```python
from build123d import *

# Parameters (mm, degrees)
BOSS_EXTRUDE1_DEPTH     = 50
CUT_EXTRUDE1_DEPTH      = 100
CUT_EXTRUDE1_DEPTH_BACK = 100
SKETCH2_R               = 2
SKETCH3_W               = 56
SKETCH3_H               = 15
BOSS_EXTRUDE2_DEPTH     = 3


with BuildPart() as part:
    # Sketch1 → Boss-Extrude1 (new, symmetric)
    with BuildSketch(Plane.XY):
        with BuildLine():
            Line((-28, 25), (-28, -10))
            Line((-28, -10), (-25, -10))
            Line((-25, -10), (-25, 0))
            Line((-25, 0), (-20, 0))
            ThreePointArc((-20, 0), (0, 20), (20, 0))
            Line((20, 0), (25, 0))
            Line((25, 0), (25, -10))
            Line((25, -10), (28, -10))
            Line((28, -10), (28, 25))
            Line((28, 25), (-28, 25))
        make_face()
    extrude(amount=BOSS_EXTRUDE1_DEPTH, both=True)

    # Sketch2 → Cut-Extrude1 (cut, two sides: drawn at the far end of the back side and taken through both)
    with BuildSketch(Plane(origin=(-25, 0, 0), x_dir=(0, 0, -1), z_dir=(1, 0, 0)).offset(-CUT_EXTRUDE1_DEPTH_BACK)):
        with Locations((-40, -5)):
            Circle(SKETCH2_R)
        with Locations((0, -5)):
            Circle(SKETCH2_R)
        with Locations((40, -5)):
            Circle(SKETCH2_R)
    extrude(amount=CUT_EXTRUDE1_DEPTH + CUT_EXTRUDE1_DEPTH_BACK, mode=Mode.SUBTRACT)

    # Sketch3 → Boss-Extrude2 (add)
    with BuildSketch(Plane.XY.offset(50)):
        with Locations((0, 17.5)):
            Rectangle(SKETCH3_W, SKETCH3_H)
    boss_extrude2 = extrude(amount=BOSS_EXTRUDE2_DEPTH)

    # Mirror1: Boss-Extrude2 across plane
    add(boss_extrude2.mirror(Plane.XY))


solid = part.part
```
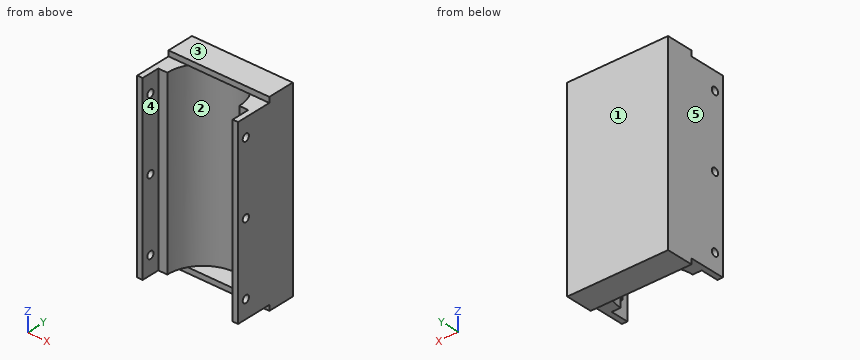
Geometry check sheet. Reference: the model listing, model coordinates, mm. Face numbers are marked on the shaded views. A direction names the side the tool comes from. Give positions to 0.01 mm unless a question says otherwise; leave off trailing zeros. Order: outer loops, then holes, each group sorted by start corner. A loop starts at its lowest first (then second) coordinate and runs counter-clockwise, first axis right, second up. Notation, with made-up numbers: (20, -8.5) - (68, -8.5) arc R27 cw to (68, 12.5) - close; hole circle Ø10 at (-4, 13.5). An arc over 180 degrees is marked (long way). Write item = value, one per line. Start each with the question number.
1) Section check A-A (z = 0). Enter the section's corners in (x, y), then the cut area to 3 significant figures.
2) Section check C-C (x = 23). Enter the section's corners in (y, z).
3) Gauge pin test, flat ends, axial feed: pin 1 Ø11.5 at (x, y) = (23.5, 2.5) entering from -Z; pin 2 Ø3.5 at (x, z) = (5, -52) entering from -Y; pin 3 Ø6.5 at (y, z) = (-5, -40) entering from +X; pin 4 Ø4 at (x, z) = (22, 12.5) entering from -Y. Record the tip position at first contact, or that the pin passes through.
4) Draft check along Z on the marked faces 1, 2 and 3. Enter one of: released by +Z, released by -Z, zero draft, split by the parting line, or undercut.
5) Section check D-D (y = 18.5). Enter the section's corners in (x, z), then the cut area to 3 significant figures.
6) Scan lines: L1, parallel to Z at x = 26.4, y = -5; L2, parallel to X at y = -1, z = 15; L3, parallel to Y at x = -27, z = 40. Record each from-to range of solid material in increasing order.
7) Access from +Z, -Z, +X, -X, +Y, -Y to the whole of each face (thin tool, end or side, straight path). Record for the marked faces 4 and 5.
8) Section check B-B (y = 7). Enter the section's corners in (x, z) (3 decimals), then the cut area to 3 significant figures.
Geometry check:
q1.outline = (-28, -10) - (-25, -10) - (-25, -7) - (-28, -7) - close; (-28, -3) - (-25, -3) - (-25, 0) - (-20, 0) arc R20 cw to (20, 0) - (25, 0) - (25, -3) - (28, -3) - (28, 25) - (-28, 25) - close; (25, -10) - (28, -10) - (28, -7) - (25, -7) - close
q1.area = 808 mm2
q2.outline = (0, -50) - (10, -50) - (10, -53) - (25, -53) - (25, 53) - (10, 53) - (10, 50) - (0, 50) - close
q3.pin_1 = -50
q3.pin_2 = 10
q3.pin_3 = 28
q3.pin_4 = 0
q4.face_1 = zero draft
q4.face_2 = undercut
q4.face_3 = released by +Z
q5.outline = (-28, -53) - (28, -53) - (28, 53) - (-28, 53) - close; hole (-7.6, -50) - (7.6, -50) - (7.6, 50) - (-7.6, 50) - close
q5.area = 4,420 mm2
q6.L1 = -50 to -42, -38 to -2, 2 to 38, 42 to 50
q6.L2 = -28 to -25, 25 to 28
q6.L3 = -10 to -7, -3 to 25
q7.face_4 = +Z, -Z, -Y
q7.face_5 = +Z, -Z, -X, +Y, -Y
q8.outline = (-28, -50) - (-18.735, -50) - (-18.735, 50) - (-28, 50) - close; (18.735, -50) - (28, -50) - (28, 50) - (18.735, 50) - close
q8.area = 1,850 mm2
